```python
from build123d import *

# Parameters (mm, degrees)
F2_R     = 5
F3_DEPTH = 8
F4_R     = 1.75
F5_DEPTH = 40
F6_R     = 4.3178383785
F7_DEPTH = 25


with BuildPart() as f1:
    # F0 (on Front) → F1 (revolve)
    with BuildSketch(Plane.XZ):
        Polygon((0.1968459624, 3.0994775003), (0, 0), (32.1352573357, -2.0408909744), (32.2620207502, -0.0449122579), (31.7640419464, 0), (32.5724625894, 8.9636184693), (33.0704413932, 8.9187062114), (33.250090425, 10.9106214268), (29.2662599942, 11.2699194904), (28.3680148353, 1.3103434133), align=None)
    revolve(axis=Axis((0.0987262279, 0, 1.554513582), (0.0633817073, 0, 0.9979893583)))

    # F2 (on face) → F3 (join)
    with BuildSketch(Plane(origin=(0.1968459624, 0, 3.0994775003), x_dir=(0.9979893583, 0, -0.0633817073), z_dir=(0.0633817073, 0, 0.9979893583))):
        Circle(F2_R)
    extrude(amount=F3_DEPTH)

    # F4 (on face) → F5 (cut)
    with BuildSketch(Plane(origin=(0.7038996206, 0, 11.0833923663), x_dir=(0.9979893583, 0, -0.0633817073), z_dir=(0.0633817073, 0, 0.9979893583))):
        Circle(F4_R)
    extrude(amount=-F5_DEPTH, mode=Mode.SUBTRACT)

    # F6 (on face) → F7 (cut)
    with BuildSketch(Plane(origin=(0.1968459624, 0, 3.0994775003), x_dir=(0.9979893583, 0, -0.0633817073), z_dir=(0.0633817073, 0, 0.9979893583))):
        Polygon((-23.8293290344, 5.2469611813), (-15.0192163679, -7.9159412247), (-8.0248648301, 6.2952913577), align=None)
        with Locations((15.0223076344, -5.7818233036)):
            Circle(F6_R)
    extrude(amount=-F7_DEPTH, mode=Mode.SUBTRACT)


solid = f1.part
```
For this review, take the finished solid that the model builds, in its own axes (mm). A direction names the side the tool comes from. Give positions to 0.01 mm unless a question says otherwise; leave off trailing zeros. Answer as a JSON object with one key per item and string values. Group by question number.
Item 1: For pin 1 Ø2 at (y, z) = (-15.5, 4.5) entering from +X; pin 2 Ø2 at (y, z) = (-14.5, 2) entering from -X; pin 3 Ø4 at (x, y) = (11, -13) entering from +Z, all flat-tipped, find the tip position at first contact; note any pin that passes through.
Item 2: For probe 1 along Y at (x, z) = (3, 10.25); probe 2 along Y at (x, z) = (-19.5, 4.5); probe 3 along Y at (x, z) = (19, 0.25), list the stretches that pass through material, from the lowest coordinate up. Write a range as [from, to].
Item 3: Draft analysis for pull direction Y (two halves, no side actions). For faces 1 (the flat face through (-6.691, 0.451, 0.425)), 2 (the cylindrical face through (30.716, 9.672, -0.935)), 3 (the cylindrical face through (-0.02, -1.71, 5.64)), 4 (the conical face through (-5.69, -27.656, 7.299)), state which applies: +Y half, -Y half, draft (parallel to the pull), parting line (faces both ways), or undercut.
Item 4: Consider section A-A on z = 10. Count the separate pieces of the cut face and the enclosed holes in it, plus the area to 3 significant figures.
Item 5: Tool access review of faces 5 (the conical face through (-5.376, -28.005, 13.465)), 6 (the flat face through (0.63, -2.15, 11.09)), 7 (the cylindrical face through (11.92, -2.86, 0.82)): name each direction out of +Z, -Z, +X, -X, +Y, -Y from which nothing blocks a thin tool from reaching the whole face with its end or side.
Check result:
{
 "1": {"pin 1": "stops at x = 28.67", "pin 2": "stops at x = -29.17", "pin 3": "stops at z = 2.54"},
 "2": {"probe 1": "y = [-31.84, -28.33], [-4.42, 4.42], [28.33, 31.84]", "probe 2": "y = [-24.84, -20.18], [20.18, 24.84]", "probe 3": "y = [-26.04, -7.58], [-3.98, 26.04]"},
 "3": {"face 1": "draft", "face 2": "parting line", "face 3": "undercut", "face 4": "undercut"},
 "4": {"separate pieces": "2", "enclosed holes": "2", "area": "768 mm^2"},
 "5": {"face 5": "+Z, +X", "face 6": "+Z", "face 7": "none"}
}
